```python
from build123d import *

# Parameters (mm, degrees)
EXTRUDE_1_DEPTH     = 10
SKETCH_6_R          = 2.1
CUT_EXTRUDE_5_DEPTH = 187.949190958
SKETCH_7_R          = 4
CUT_EXTRUDE_6_DEPTH = 1
FILLET_1_R          = 3
SKETCH_8_R          = 4.25
CUT_EXTRUDE_7_DEPTH = 10


with BuildPart() as part:
    # 草图5 → 凸台-拉伸1 (new body)
    with BuildSketch(Plane.XY):
        Polygon((0, 0), (0, 175), (44, 175), (44, 125), (65, 35), (65, 0), align=None)
    extrude(amount=EXTRUDE_1_DEPTH)

    # 草图6 → 切除-拉伸5 (cut, through all)
    with BuildSketch(Plane.XY.offset(10)):
        with Locations((15, 163)):
            Circle(SKETCH_6_R)
        with Locations((15, 109)):
            Circle(SKETCH_6_R)
    extrude(amount=-CUT_EXTRUDE_5_DEPTH, mode=Mode.SUBTRACT)

    # 草图7 → 切除-拉伸6 (cut)
    with BuildSketch(Plane.XY.offset(10)):
        with Locations((15, 163)):
            Circle(SKETCH_7_R)
        with Locations((15, 109)):
            Circle(SKETCH_7_R)
    extrude(amount=-CUT_EXTRUDE_6_DEPTH, mode=Mode.SUBTRACT)

    # 圆角1
    fillet_1_edges = [part.edges().sort_by_distance(p)[0] for p in [
        (0, 0, 5),
        (44, 175, 5),
        (44, 125, 5),
    ]]
    fillet(fillet_1_edges, radius=FILLET_1_R)

    # 草图8 → 切除-拉伸7 (cut)
    with BuildSketch(Plane.XY.offset(10)):
        with Locations((15, 136)):
            Circle(SKETCH_8_R)
    extrude(amount=-CUT_EXTRUDE_7_DEPTH, mode=Mode.SUBTRACT)


solid = part.part
```
Read the model definition and answer for the solid it produces. Units are mm, in the model's axes. A direction names the side the tool comes from. Round coordinates to 2 decimals unless told otherwise and drop trailing zeros. Write each loop counter-clockwise with the first axis right and the second up, starting at its lowest first coordinate (ties: lowest second). Pieces come first, ordered by that corner, then holes. Notation, with made-up numbers: (-7.75, 26) -> (15.25, 26) arc R13 cw to (15.25, 36) -> close; hole circle Ø10 at (13, 53). An arc over 180 degrees is marked (long way). Answer in a Markdown table with one row per item. Add a question column.
1) Find section A-A, the plane y = 136. Determine the outline of the cut face in (x, z), and give its area (3 significant figures).
2) Find section C-C, the plane z = 4.25. Determine the outline of the cut face in (x, y).
3) Given P1, Ø4, axis at y = 69.5, z = 9, coming from the +X side; P2, Ø5, axis at y = 58, z = 7, coming from the +X side; P3, Ø4, axis at x = 14, y = 110.5, coming from the +Z side, each flat-ended and moving along its own axis, determine where each tip first touches the part or whether it passes through.
4) Consider line 1 (Y direction, x = 15, z = 9.65); line 2 (Y direction, x = 15, z = 5.25); line 3 (X direction, y = 147, z = 4.75). Determine where each line is inside the solid, lowest interval first.
5) Find section D-D, the plane y = 109. Determine the outline of the cut face in (x, z), and give its area (3 significant figures).
6) Determine the mould class of faces 4 (the face through (34, 0, 5)), 5 (the face through (65, 18, 5)), 6 (the face through (14.54, 106.95, 4.56)) for opening direction X: pulls with the +X half, pulls with the -X half, needs draft (parallel to the pull), parting line crosses it, or undercut.
7) Which of the six approach directions +Z, -Z, +X, -X, +Y, -Y give full straight-line access (tool end or side, diameter ignored) to faces 1 (the face through (44, 149, 5)), 2 (the face through (17, 161, 9)), 3 (the face through (0, 88, 5))?
8) Find section B-B, the plane x = 15. Determine the outline of the cut face in (y, z), and give its area (3 significant figures).
Findings below:
| question | item | result |
|---|---|---|
| 1 | outline | (0, 0) -> (10.75, 0) -> (10.75, 10) -> (0, 10) -> close; (19.25, 0) -> (44, 0) -> (44, 10) -> (19.25, 10) -> close |
| 1 | area | 355 mm² |
| 2 | outline | (0, 3) arc R3 ccw to (3, 0) -> (65, 0) -> (65, 35) -> (44.08, 124.66) arc R3 cw to (44, 125.35) -> (44, 172) arc R3 ccw to (41, 175) -> (0, 175) -> close; hole circle Ø8.5 at (15, 136); hole circle Ø4.2 at (15, 109); hole circle Ø4.2 at (15, 163) |
| 3 | P1 | x = 57.42 |
| 3 | P2 | x = 60.22 |
| 3 | P3 | z = 9 |
| 4 | line 1 | 0 to 105, 113 to 131.75, 140.25 to 159, 167 to 175 |
| 4 | line 2 | 0 to 106.9, 111.1 to 131.75, 140.25 to 160.9, 165.1 to 175 |
| 4 | line 3 | 0 to 44 |
| 5 | outline | (0, 0) -> (12.9, 0) -> (12.9, 9) -> (11, 9) -> (11, 10) -> (0, 10) -> close; (17.1, 0) -> (47.73, 0) -> (47.73, 10) -> (19, 10) -> (19, 9) -> (17.1, 9) -> close |
| 5 | area | 432 mm² |
| 6 | face 4 | needs draft |
| 6 | face 5 | pulls with the +X half |
| 6 | face 6 | undercut |
| 7 | face 1 | +Z, -Z, +X, +Y |
| 7 | face 2 | +Z |
| 7 | face 3 | +Z, -Z, -X, +Y, -Y |
| 8 | outline | (0, 0) -> (106.9, 0) -> (106.9, 9) -> (105, 9) -> (105, 10) -> (0, 10) -> close; (111.1, 0) -> (131.75, 0) -> (131.75, 10) -> (113, 10) -> (113, 9) -> (111.1, 9) -> close; (140.25, 0) -> (160.9, 0) -> (160.9, 9) -> (159, 9) -> (159, 10) -> (140.25, 10) -> close; (165.1, 0) -> (175, 0) -> (175, 10) -> (167, 10) -> (167, 9) -> (165.1, 9) -> close |
| 8 | area | 1,570 mm² |
